from build123d import *

# Parameters (mm, degrees)
SKETCH1_W           = 90
SKETCH1_H           = 14
SKETCH1_R           = 2
SKETCH1_R_2         = 3.5
BOSS_EXTRUDE1_DEPTH = 4
SKETCH2_W           = 14
SKETCH2_H           = 14
BOSS_EXTRUDE2_DEPTH = 2
SKETCH3_W           = 12
SKETCH3_H           = 12
BOSS_EXTRUDE3_DEPTH = 6
SKETCH4_W           = 14
SKETCH4_H           = 14
BOSS_EXTRUDE4_DEPTH = 9
SKETCH5_W           = 2
SKETCH5_H           = 10
BOSS_EXTRUDE5_DEPTH = 2
SKETCH6_R           = 2
CUT_EXTRUDE1_DEPTH  = 9
SKETCH8_R           = 4
SKETCH8_R_2         = 2
CUT_EXTRUDE2_DEPTH  = 48.095647357
CHAMFER1_SIZE       = 2
CHAMFER2_SIZE       = 2


with BuildPart() as part:
    # Sketch1 → Boss-Extrude1 (new body)
    # profile 1 of 2: a face of its own
    with BuildSketch(Plane(origin=(0, 0, 0), x_dir=(1, 0, 0), z_dir=(0, 1, 0))):
        Rectangle(SKETCH1_W, SKETCH1_H)
        Circle(SKETCH1_R, mode=Mode.SUBTRACT)
        with Locations(Location((38, 0, 0), (0, 0, 270))):
            Circle(SKETCH1_R_2, mode=Mode.SUBTRACT)
        with Locations(Location((-38, 0, 0), (0, 0, 270))):
            Circle(SKETCH1_R_2, mode=Mode.SUBTRACT)
    # profile 2 of 2: a face of its own
    with BuildSketch(Plane(origin=(0, 0, 0), x_dir=(1, 0, 0), z_dir=(0, 1, 0))):
        Circle(SKETCH1_R)
    extrude(amount=BOSS_EXTRUDE1_DEPTH)

    # Sketch2 → Boss-Extrude2 (add)
    with BuildSketch(Plane(origin=(0, 4, 0), x_dir=(1, 0, 0), z_dir=(0, 1, 0))):
        Rectangle(SKETCH2_W, SKETCH2_H)
    extrude(amount=BOSS_EXTRUDE2_DEPTH)

    # Sketch3 → Boss-Extrude3 (add)
    with BuildSketch(Plane(origin=(0, 6, 0), x_dir=(1, 0, 0), z_dir=(0, 1, 0))):
        Rectangle(SKETCH3_W, SKETCH3_H)
    extrude(amount=BOSS_EXTRUDE3_DEPTH)

    # Sketch4 → Boss-Extrude4 (add)
    with BuildSketch(Plane(origin=(0, 12, 0), x_dir=(1, 0, 0), z_dir=(0, 1, 0))):
        Rectangle(SKETCH4_W, SKETCH4_H)
    extrude(amount=BOSS_EXTRUDE4_DEPTH)

    # Sketch5 → Boss-Extrude5 (add)
    with BuildSketch(Plane(origin=(0, 21, 0), x_dir=(1, 0, 0), z_dir=(0, 1, 0))):
        with Locations((-6, 0)):
            Rectangle(SKETCH5_W, SKETCH5_H)
        with Locations((6, 0)):
            Rectangle(SKETCH5_W, SKETCH5_H)
    extrude(amount=BOSS_EXTRUDE5_DEPTH)

    # Sketch6 → Cut-Extrude1 (cut)
    with BuildSketch(Plane(origin=(0, 21, 0), x_dir=(1, 0, 0), z_dir=(0, 1, 0))):
        with Locations(Location((0, 0, 0), (0, 0, 270))):
            Circle(SKETCH6_R)
    extrude(amount=-CUT_EXTRUDE1_DEPTH, mode=Mode.SUBTRACT)

    # Sketch8 → Cut-Extrude2 (cut, through all)
    # profile 1 of 2: a face of its own
    with BuildSketch(Plane(origin=(0, 12, 0), x_dir=(1, 0, 0), z_dir=(0, 1, 0))):
        with Locations(Location((0, 0, 0), (0, 0, 270))):
            Circle(SKETCH8_R)
        with Locations(Location((0, 0, 0), (0, 0, 270))):
            Circle(SKETCH8_R_2, mode=Mode.SUBTRACT)
    # profile 2 of 2: a face of its own
    with BuildSketch(Plane(origin=(0, 12, 0), x_dir=(1, 0, 0), z_dir=(0, 1, 0))):
        with Locations(Location((0, 0, 0), (0, 0, 270))):
            Circle(SKETCH8_R_2)
    extrude(amount=-CUT_EXTRUDE2_DEPTH, mode=Mode.SUBTRACT)

    # Chamfer1
    chamfer1_edges = [part.edges().sort_by_distance(p)[0] for p in [
        (7, 5, 7),
        (6, 9, 6),
        (7, 16.5, 7),
        (7, 16.5, -7),
        (7, 5, -7),
        (-7, 5, 7),
        (-7, 5, -7),
        (-6, 9, -6),
        (-6, 9, 6),
        (-7, 16.5, 7),
        (45, 2, 7),
        (-45, 2, 7),
        (-45, 2, -7),
        (45, 2, -7),
        (-7, 16.5, -7),
    ]]
    chamfer(chamfer1_edges, length=CHAMFER1_SIZE - 0.0001)  # a hair under: the kernel refuses the full size

    # Chamfer2
    chamfer2_edges = [part.edges().sort_by_distance(p)[0] for p in [
        (0, 12, -2),
    ]]
    chamfer(chamfer2_edges, length=CHAMFER2_SIZE - 0.0001)  # a hair under: the kernel refuses the full size


solid = part.part
Can you work these out from the model? Positions are in its coordinate system, mm. A direction names the side the tool comes from. Coordinates: 2 decimals unless noted, no trailing zeros. Loops run counter-clockwise (first coordinate to the right, second up) from the corner with the lowest first, then second, coordinate; pieces in that order, holes last. Notation, with made-up numbers: M 49,83.25 L 101,83.25 A24 ccw 101,101.25 Z; hole C 71,61.25 d3. An arc over 180 degrees is marked long. Return JSON: item names as keys, results as strings. Group by question number.
Item 1: I'm going to push flat-ended pins straight in: pin 1 Ø8 at (y, z) = (15, 1) entering from -X; pin 2 Ø8 at (x, z) = (24, -5.5) entering from +Y; pin 3 Ø4 at (x, z) = (-38, 0) entering from -Y; pin 4 Ø3 at (x, y) = (1, 8) entering from +Z. Where does each tip first touch, or does it pass through?
Item 2: Imagine slicing it at C-C (z = 0). Give the number of separate pieces and of enclosed holes in the cut face, and give its area (3 significant figures).
Item 3: Imagine slicing it at B-B (y = 19.5). Please give me the cut outline in (x, z).
Item 4: If I drill on L1, parallel to X at y = 0.85, z = 0; L2, parallel to Y at x = 10, z = -3; L3, parallel to X at y = 21.75, z = -4.25, over which ranges is the centre line in solid material (lowest first)? Write a range as from..to.
Item 5: Imagine slicing it at A-A (x = -38). Please give me the cut outline in (y, z).
Item 6: On a 3-axis mill with a long thin cutter (end or side, diameter ignored), from which of +Z, -Z, +X, -X, +Y, -Y can I reach the whole of each face in a straight line? I mean faces 1 (the flat face through (6, 5, -6)), 2 (the flat face through (-5, 9, 5)), 3 (the flat face through (6, 22, -5)). Say none if no direction works.
Verdict:
{
 "1": {"pin 1": "stops at x = -7", "pin 2": "stops at y = 4", "pin 3": "passes through", "pin 4": "stops at z = 6"},
 "2": {"separate pieces": "4", "enclosed holes": "0", "area": "402 mm^2"},
 "3": {"outline": "M -7,-5 L -5,-7 L 5,-7 L 7,-5 L 7,5 L 5,7 L -5,7 L -7,5 Z; hole C 0,0 d4"},
 "4": {"L1": "x = -45..-41.5, -34.5..-4, 4..34.5, 41.5..45", "L2": "y = 0..4", "L3": "x = -7..-5, 5..7"},
 "5": {"outline": "M 0,-7 L 4,-7 L 4,-3.5 L 0,-3.5 Z; M 0,3.5 L 4,3.5 L 4,7 L 0,7 Z"},
 "6": {"face 1": "-Z, +X, +Y", "face 2": "+Z, -X", "face 3": "-Z, +X, -X, +Y"}
}
